```python
from build123d import *

# Parameters (mm, degrees)
SKETCH1_W           = 20
SKETCH1_H           = 40
BOSS_EXTRUDE1_DEPTH = 5
SKETCH2_W           = 20
SKETCH2_H           = 9.75
BOSS_EXTRUDE2_DEPTH = 10
SKETCH3_R           = 1.75
CUT_EXTRUDE1_DEPTH  = 5
SKETCH4_R           = 3.363406012
CUT_EXTRUDE2_DEPTH  = 3
SKETCH5_R           = 1.75
CUT_EXTRUDE3_DEPTH  = 8
SKETCH6_W           = 6
SKETCH6_H           = 10
CUT_EXTRUDE4_DEPTH  = 3
SKETCH7_R           = 1.75
CUT_EXTRUDE5_DEPTH  = 3
FILLET1_R           = 5
SKETCH10_W          = 11.5
SKETCH10_H          = 5
CUT_EXTRUDE6_DEPTH  = 2


with BuildPart() as part:
    # Sketch1 → Boss-Extrude1 (new body)
    with BuildSketch(Plane(origin=(0, 0, 0), x_dir=(1, 0, 0), z_dir=(0, 1, 0))):
        Rectangle(SKETCH1_W, SKETCH1_H)
    extrude(amount=BOSS_EXTRUDE1_DEPTH)

    # Sketch2 → Boss-Extrude2 (add)
    with BuildSketch(Plane.XZ):
        with Locations((0, 15.125)):
            Rectangle(SKETCH2_W, SKETCH2_H)
        with Locations((0, -15.125)):
            Rectangle(SKETCH2_W, SKETCH2_H)
    extrude(amount=BOSS_EXTRUDE2_DEPTH)

    # Sketch3 → Cut-Extrude1 (cut)
    with BuildSketch(Plane(origin=(0, 5, 0), x_dir=(1, 0, 0), z_dir=(0, 1, 0))):
        with Locations(Location((-7.5, -8, 0), (0, 0, 270))):
            Circle(SKETCH3_R)
        with Locations(Location((-7.5, 8, 0), (0, 0, 270))):
            Circle(SKETCH3_R)
        with Locations(Location((7.5, -8, 0), (0, 0, 270))):
            Circle(SKETCH3_R)
        with Locations(Location((7.5, 8, 0), (0, 0, 270))):
            Circle(SKETCH3_R)
    extrude(amount=-CUT_EXTRUDE1_DEPTH, mode=Mode.SUBTRACT)

    # Sketch4 → Cut-Extrude2 (cut)
    with BuildSketch(Plane.XZ):
        with Locations((7.5, 8)):
            Circle(SKETCH4_R)
        with Locations((-7.5, 8)):
            Circle(SKETCH4_R)
        with Locations((-7.5, -8)):
            Circle(SKETCH4_R)
        with Locations((7.5, -8)):
            Circle(SKETCH4_R)
    extrude(amount=-CUT_EXTRUDE2_DEPTH, mode=Mode.SUBTRACT)

    # Sketch5 → Cut-Extrude3 (cut)
    with BuildSketch(Plane.XZ.offset(10)):
        with Locations(Location((-5, -15, 0), (0, 0, 270))):
            Circle(SKETCH5_R)
        with Locations(Location((5, -15, 0), (0, 0, 270))):
            Circle(SKETCH5_R)
        with Locations(Location((-5, 15, 0), (0, 0, 270))):
            Circle(SKETCH5_R)
        with Locations(Location((5, 15, 0), (0, 0, 270))):
            Circle(SKETCH5_R)
    extrude(amount=-CUT_EXTRUDE3_DEPTH, mode=Mode.SUBTRACT)

    # Sketch6 → Cut-Extrude4 (cut)
    with BuildSketch(Plane.XZ.offset(2)):
        with Locations((-5, -15)):
            Rectangle(SKETCH6_W, SKETCH6_H)
        with Locations((5, -15)):
            Rectangle(SKETCH6_W, SKETCH6_H)
        with Locations((5, 15)):
            Rectangle(SKETCH6_W, SKETCH6_H)
        with Locations((-5, 15)):
            Rectangle(SKETCH6_W, SKETCH6_H)
    extrude(amount=CUT_EXTRUDE4_DEPTH, mode=Mode.SUBTRACT)

    # Sketch7 → Cut-Extrude5 (cut)
    with BuildSketch(Plane.XZ.offset(2)):
        with Locations(Location((-5, -15, 0), (0, 0, 270))):
            Circle(SKETCH7_R)
        with Locations(Location((5, -15, 0), (0, 0, 270))):
            Circle(SKETCH7_R)
        with Locations(Location((5, 15, 0), (0, 0, 270))):
            Circle(SKETCH7_R)
        with Locations(Location((-5, 15, 0), (0, 0, 270))):
            Circle(SKETCH7_R)
    extrude(amount=-CUT_EXTRUDE5_DEPTH, mode=Mode.SUBTRACT)

    # Fillet1
    # the kernel refuses this fillet: 5 mm, written as the material it takes off along each edge
    with BuildSketch(Plane(origin=(-10, 17.5, -20), x_dir=(0, 0, 1), z_dir=(0, -1, 0)), Plane(origin=(10, -22.5, -20), x_dir=(0, 0, 1), z_dir=(0, 1, 0)), Plane(origin=(-10, 17.5, 20), x_dir=(1, 0, 0), z_dir=(0, -1, 0)), Plane(origin=(10, -22.5, 20), x_dir=(-1, 0, 0), z_dir=(0, 1, 0))) as fillet1_piece_1:
        with BuildLine():
            CenterArc((FILLET1_R, -FILLET1_R), FILLET1_R, 90, 90)
            Line((0, -FILLET1_R), (0, 0))
            Line((0, 0), (FILLET1_R, 0))
        make_face()
    extrude(amount=40, mode=Mode.SUBTRACT)

    # Sketch10 → Cut-Extrude6 (cut)
    with BuildSketch(Plane(origin=(10, 0, 0), x_dir=(0, 0, -1), z_dir=(1, 0, 0))):
        with Locations((0, 2.5)):
            Rectangle(SKETCH10_W, SKETCH10_H)
    extrude(amount=-CUT_EXTRUDE6_DEPTH, mode=Mode.SUBTRACT)


solid = part.part
```
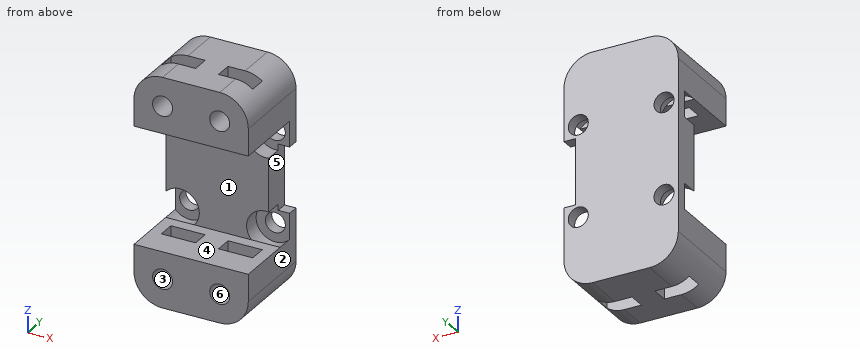
For this review, take the finished solid that the model builds, in its own axes (mm). Face numbers are marked on the shaded views. A direction names the side the tool comes from. Give positions to 0.01 mm unless a question says otherwise; leave off trailing zeros. Write each loop counter-clockwise with the first axis right and the second up, starting at its lowest first coordinate (ties: lowest second). Pieces come first, ordered by that corner, then holes. Notation, with made-up numbers: M 55.5,5 L 63.5,5 A17 ccw 63.5,32 Z; hole C 71,52 d3. An arc over 180 degrees is marked long. Answer as CSV lines item,"result".
1. Consider section A-A, the plane y = 3.5. Write out the cut boundary in (x, z).
Findings:
outline,"M -10,-15 A5 ccw -5,-20 L 5,-20 A5 ccw 10,-15 L 10,-5.75 L 8,-5.75 L 8,5.75 L 10,5.75 L 10,15 A5 ccw 5,20 L -5,20 A5 ccw -10,15 Z; hole C -7.5,-8 d3.5; hole C -7.5,8 d3.5; hole C 7.5,-8 d3.5; hole C 7.5,8 d3.5"
2. Draft analysis for pull direction X (two halves, no side actions). For the marked faces 1, 2 and 3, state which applies: +X half, -X half, draft (parallel to the pull), parting line (faces both ways), or undercut.
Findings:
face 1,"draft"
face 2,"+X half"
face 3,"undercut"
3. Consider section B-B, the plane x = 2.5. Write out the cut boundary in (y, z), then the cut area to 4 significant figures.
Findings:
outline,"M -10,-20 L -5,-20 L -5,-10.25 L -10,-10.25 Z; M -10,10.25 L -5,10.25 L -5,20 L -10,20 Z; M -2,-20 L 5,-20 L 5,20 L -2,20 L -2,10.25 L 0,10.25 L 0,-10.25 L -2,-10.25 Z"
area,"336.5 mm2"
4. Consider section C-C, the plane y = -2.75. Write out the cut boundary in (x, z), then the cut area to 3 significant figures.
Findings:
outline,"M -10,-15 A5 ccw -8,-19 L -8,-10.25 L -10,-10.25 Z; M -10,10.25 L -8,10.25 L -8,19 A5 ccw -10,15 Z; M -2,-20 L 2,-20 L 2,-10.25 L -2,-10.25 Z; M -2,10.25 L 2,10.25 L 2,20 L -2,20 Z; M 8,-19 A5 ccw 10,-15 L 10,-10.25 L 8,-10.25 Z; M 8,10.25 L 10,10.25 L 10,15 A5 ccw 8,19 Z"
area,"138 mm2"
5. Wall thickness on line 1 (X direction, y = 3.9, z = 8); line 2 (X direction, y = -2.5, z = -12); line 3 (Y direction, x = 4, z = -12.5): over which ranges is each line inside the solid? List them lowest first.
Findings:
line 1,"x = -10 to -9.25, -5.75 to 5.75, 9.25 to 10"
line 2,"x = -10 to -8, -2 to 2, 8 to 10"
line 3,"y = -10 to -5, -2 to 5"
6. For the marked faces 4, 5 and 6, list the 3-axis set-ups (+Z, -Z, +X, -X, +Y, -Y) from which the entire face can be reached by the end or side of a thin tool; tool diameter is ignored.
Findings:
face 4,"+X, -X, -Y"
face 5,"+X, +Y, -Y"
face 6,"-Y"
7. Consider section D-D, the plane z = 8. Write out the cut boundary in (x, y).
Findings:
outline,"M -10,3 L -9.25,3 L -9.25,5 L -10,5 Z; M -5.75,3 L -4.14,3 L -4.14,0 L 4.14,0 L 4.14,3 L 5.75,3 L 5.75,5 L -5.75,5 Z; M 9.25,3 L 10,3 L 10,5 L 9.25,5 Z"
8. For pin 1 (12 mm diameter, centred on x = 6, z = 9, fed in from -Y); pin 2 (12 mm diameter, centred on x = 7.5, z = 2.5, fed in from -Y); pin 3 (3 mm diameter, centred on x = 7, z = 8, fed in from -Y); pin 4 (5.5 mm diameter, centred on y = 1.5, z = -1, fed in from +X), all flat-tipped, find the tip position at first contact; note any pin that passes through.
Findings:
pin 1,"stops at y = -10"
pin 2,"stops at y = 0"
pin 3,"stops at y = 3"
pin 4,"stops at x = 8"
